Source: three-view drawing plus pictorial views. Frame: mm from the lowest corner of the part. A direction names the side the tool comes from. Round coordinates to 2 decimals unless told otherwise and drop trailing zeros. Loops run counter-clockwise (first coordinate to the right, second up) from the corner with the lowest first, then second, coordinate; pieces in that order, holes last. Notation, with made-up numbers: (9.5, -5.75) -> (39.5, -5.75) arc R18 ccw to (39.5, 28.25) -> close; hole circle Ø10 at (74, -20). An arc over 180 degrees is marked (long way). Answer as a JSON object with one key per item and string values. Group by question number.
Item 1: Section query B-B on x = 45.4. Return loops of the section in (y, z), and give its area (3 significant figures).
Item 2: Set-up query: the marked faces 1, 2 and 3. Return all of +Z, -Z, +X, -X, +Y, -Y with unobstructed straight access to the full face (end or side cutting, diameter ignored); none if empty.
Item 3: Pin query (flat end, axial travel): pin 1 (1.7 mm diameter, centred on x = 14.5, z = 1.5, fed in from -Y); pin 2 (6 mm diameter, centred on x = 39.5, z = 48, fed in from -Y); pin 3 (3.5 mm diameter, centred on x = 34.1, z = 31.3, fed in from +Y); pin 4 (16.5 mm diameter, centred on y = 36, z = 5.5, fed in from -X). Return the tip coordinate at first contact, or that it passes through.
Item 4: Draft query along Y for the marked faces 4, 5, 6 and 7. Return one class per face: released by +Y, released by -Y, zero draft, split by the parting line, or undercut.
Item 5: Section query D-D on y = 28. Return loops of the section in (x, z).
Item 6: Section query C-C on x = 35. Return loops of the section in (y, z), and give its area (3 significant figures).
Item 7: Material intervals for line 1 (Z direction, x = 34.1, y = 68.8); line 2 (X direction, y = 68, z = 39) (1 decimal); line 3 (Y direction, x = 18.5, z = 60.5), sorted ascending. Write a range as [from, to].
Item 8: Section query A-A on z = 39.8. Return loops of the section in (x, y).
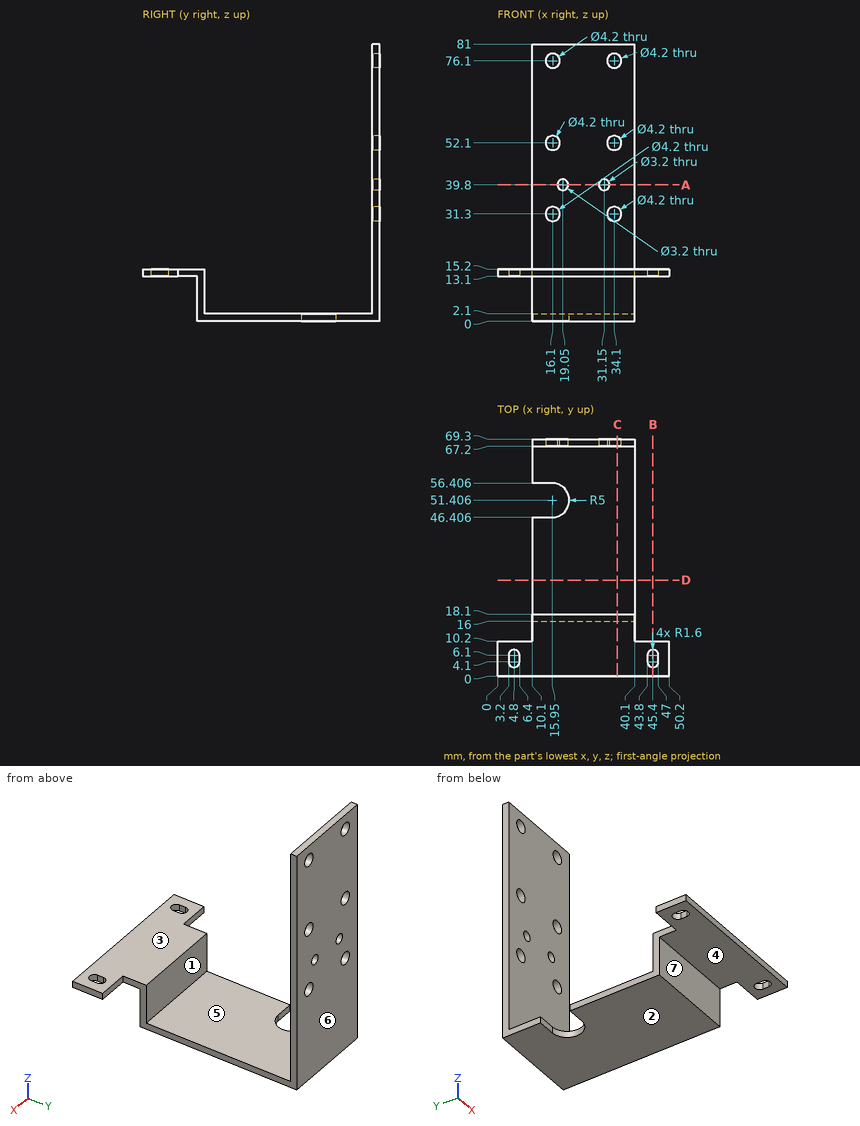
Solved:
{
 "1": {"outline": "(0, 13.1) -> (2.5, 13.1) -> (2.5, 15.2) -> (0, 15.2) -> close; (7.7, 13.1) -> (10.2, 13.1) -> (10.2, 15.2) -> (7.7, 15.2) -> close", "area": "10.5 mm²"},
 "2": {"face 1": "+Z, +X, -X", "face 2": "-Z, +X, -X, +Y, -Y", "face 3": "+Z, +X, -X, -Y"},
 "3": {"pin 1": "y = 16", "pin 2": "y = 67.2", "pin 3": "through", "pin 4": "x = 10.1"},
 "4": {"face 4": "zero draft", "face 5": "undercut", "face 6": "released by +Y", "face 7": "released by -Y"},
 "5": {"outline": "(10.1, 0) -> (40.1, 0) -> (40.1, 2.1) -> (10.1, 2.1) -> close"},
 "6": {"outline": "(0, 13.1) -> (16, 13.1) -> (16, 0) -> (69.3, 0) -> (69.3, 29.4) -> (67.2, 29.4) -> (67.2, 2.1) -> (18.1, 2.1) -> (18.1, 15.2) -> (0, 15.2) -> close; (67.2, 33.2) -> (69.3, 33.2) -> (69.3, 50.2) -> (67.2, 50.2) -> close; (67.2, 54) -> (69.3, 54) -> (69.3, 74.2) -> (67.2, 74.2) -> close; (67.2, 78) -> (69.3, 78) -> (69.3, 81) -> (67.2, 81) -> close", "area": "315 mm²"},
 "7": {"line 1": "[0, 29.2], [33.4, 50], [54.2, 74], [78.2, 81]", "line 2": "[10.1, 17.7], [20.4, 29.8], [32.5, 40.1]", "line 3": "[67.2, 69.3]"},
 "8": {"outline": "(10.1, 67.2) -> (17.45, 67.2) -> (17.45, 69.3) -> (10.1, 69.3) -> close; (20.65, 67.2) -> (29.55, 67.2) -> (29.55, 69.3) -> (20.65, 69.3) -> close; (32.75, 67.2) -> (40.1, 67.2) -> (40.1, 69.3) -> (32.75, 69.3) -> close"}
}
